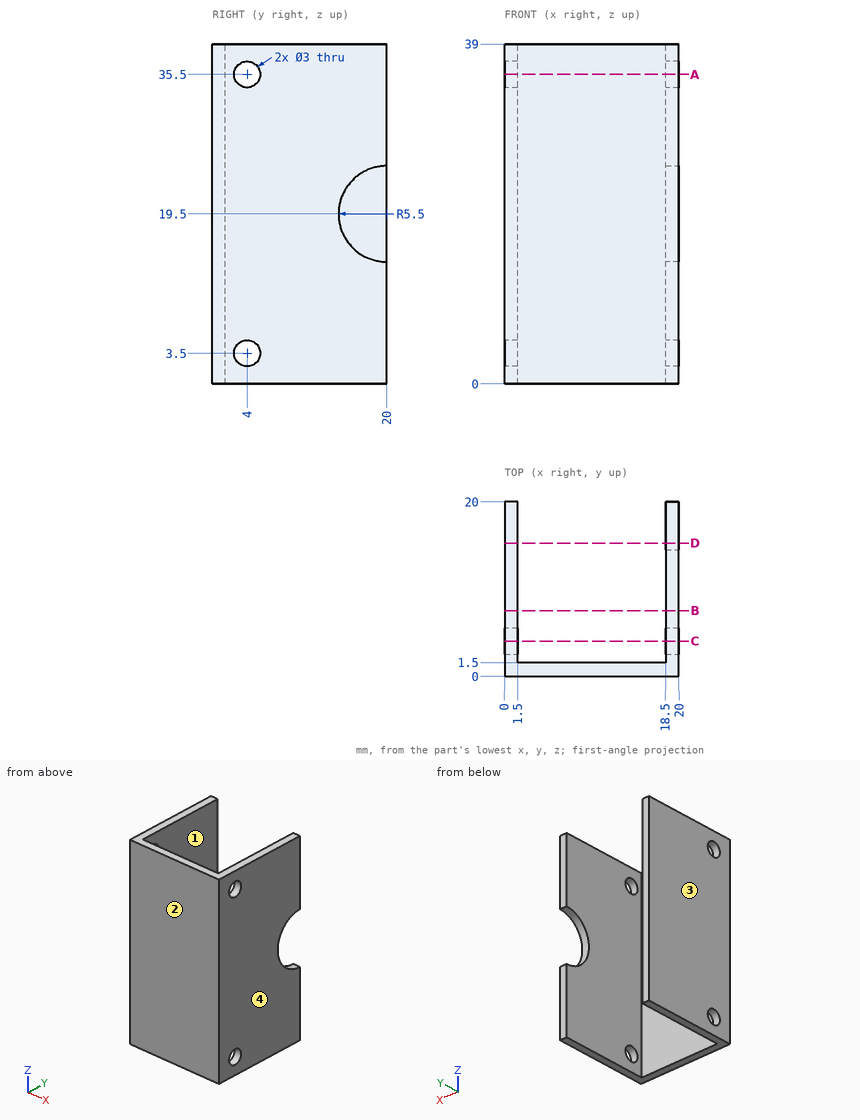
The figure shows three views and two pictorial views of one solid part (mm, origin at its lowest corner). Answer the questions. Round coordinates to 2 decimals unless told otherwise and drop trailing zeros. Loops run counter-clockwise (first coordinate to the right, second up) from the corner with the lowest first, then second, coordinate; pieces in that order, holes last. Notation, with made-up numbers: M -10,41.5 L 44,41.5 A15 cw 44,65.5 Z; hole C 52.25,-27.5 d11. An arc over 180 degrees is marked long. Return JSON: item names as keys, results as strings.
Q1. Find section D-D, the plane y = 15.25. Determine the outline of the cut face in (x, z), plus the area to 3 significant figures.
Results list:
{"outline": "M 0,0 L 1.5,0 L 1.5,39 L 0,39 Z; M 18.5,0 L 20,0 L 20,16.73 L 18.5,16.73 Z; M 18.5,22.27 L 20,22.27 L 20,39 L 18.5,39 Z", "area": "109 mm2"}
Q2. Find section C-C, the plane y = 4. Determine the outline of the cut face in (x, z), plus the area to 3 significant figures.
Results list:
{"outline": "M 0,0 L 1.5,0 L 1.5,2 L 0,2 Z; M 0,5 L 1.5,5 L 1.5,34 L 0,34 Z; M 0,37 L 1.5,37 L 1.5,39 L 0,39 Z; M 18.5,0 L 20,0 L 20,2 L 18.5,2 Z; M 18.5,5 L 20,5 L 20,34 L 18.5,34 Z; M 18.5,37 L 20,37 L 20,39 L 18.5,39 Z", "area": "99.0 mm2"}
Q3. The mould has two halves that part along X. Classify the marked faces 1, 2, 3 and 4: released by +X, released by -X, zero draft, split by the parting line, or undercut.
Results list:
{"face 1": "undercut", "face 2": "zero draft", "face 3": "released by -X", "face 4": "released by +X"}
Q4. Find section A-A, the plane z = 35.5. Determine the outline of the cut face in (x, y).
Results list:
{"outline": "M 0,0 L 20,0 L 20,2.5 L 18.5,2.5 L 18.5,1.5 L 1.5,1.5 L 1.5,2.5 L 0,2.5 Z; M 0,5.5 L 1.5,5.5 L 1.5,20 L 0,20 Z; M 18.5,5.5 L 20,5.5 L 20,20 L 18.5,20 Z"}
Q5. Each of these flat-tipped pins is pushed along its axis until it touches: pin 1 Ø2.5 at (y, z) = (4, 35.5) entering from -X; pin 2 Ø5.5 at (y, z) = (9, 21.5) entering from -X; pin 3 Ø4 at (x, z) = (11, 7) entering from +Y. Where does it stop, or does it pass through?
Results list:
{"pin 1": "passes through", "pin 2": "stops at x = 0", "pin 3": "stops at y = 1.5"}
Q6. Find section B-B, the plane y = 7.5. Determine the outline of the cut face in (x, z), plus the area to 3 significant figures.
Results list:
{"outline": "M 0,0 L 1.5,0 L 1.5,39 L 0,39 Z; M 18.5,0 L 20,0 L 20,39 L 18.5,39 Z", "area": "117 mm2"}
Q7. Find the intervals of material crossed by line 1 along Z through (x, y) = (18.9, 4); line 2 along X through (y, z) = (11.25, 37); line 3 along Y through (x, z) = (17.25, 23), in increasing order. Write a range as from..to.
Results list:
{"line 1": "z = 0..2, 5..34, 37..39", "line 2": "x = 0..1.5, 18.5..20", "line 3": "y = 0..1.5"}
